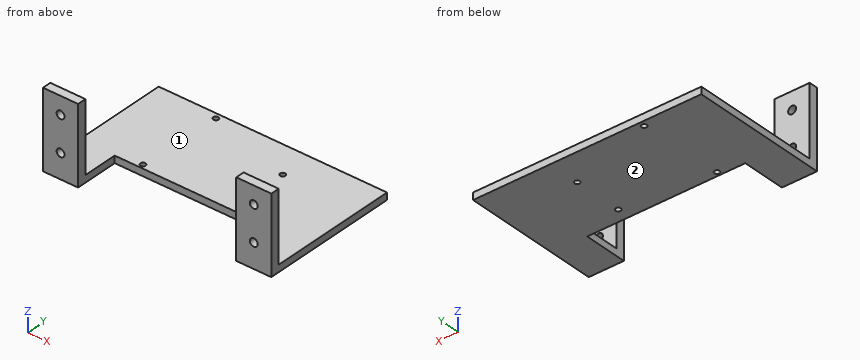
from build123d import *

# Parameters (mm, degrees)
SKETCH1_W                 = 20
SKETCH1_H                 = 44
SKETCH1_R                 = 2.25
BOSS_EXTRUDE1_DEPTH       = 5
BOSS_EXTRUDE1_2_DEPTH     = 5
SKETCH2_W                 = 130.04
SKETCH2_H                 = 4
BOSS_EXTRUDE2_DEPTH       = 74
BOSS_EXTRUDE2_DEPTH_BACK  = 5
SKETCH3_W                 = 90.04
SKETCH3_H                 = 25
CUT_EXTRUDE1_DEPTH        = 5
F_3_0MM_DOWEL_HOLE1_D     = 3
F_3_0MM_DOWEL_HOLE1_DEPTH = 5
F_3_0MM_DOWEL_HOLE1_TIP   = 0.901290929


with BuildPart() as part:
    # Sketch1 → Boss-Extrude1 (new body)
    with BuildSketch(Plane(origin=(0, 0, 0), x_dir=(1, 0, 0), z_dir=(0, 1, 0))):
        with Locations((0, 12)):
            Rectangle(SKETCH1_W, SKETCH1_H)
        Circle(SKETCH1_R, mode=Mode.SUBTRACT)
        with Locations((0, 20)):
            Circle(SKETCH1_R, mode=Mode.SUBTRACT)
    extrude(amount=BOSS_EXTRUDE1_DEPTH)



with BuildPart() as body_2:
    # Sketch1 → Boss-Extrude1 2 (new body)
    with BuildSketch(Plane(origin=(0, 0, 0), x_dir=(1, 0, 0), z_dir=(0, 1, 0))):
        with Locations((110.04, 12)):
            Rectangle(SKETCH1_W, SKETCH1_H)
        with Locations((110.04, 20)):
            Circle(SKETCH1_R, mode=Mode.SUBTRACT)
        with Locations((110.04, 0)):
            Circle(SKETCH1_R, mode=Mode.SUBTRACT)
    extrude(amount=BOSS_EXTRUDE1_2_DEPTH)


with BuildPart() as part_1:
    add(part.part)

    add(body_2.part)  # Boss-Extrude2 merges body 2
    # Sketch2 → Boss-Extrude2 (add, two sides)
    with BuildSketch(Plane(origin=(0, 5, 0), x_dir=(1, 0, 0), z_dir=(0, 1, 0))) as boss_extrude2_sk:
        with Locations((55.02, 32)):
            Rectangle(SKETCH2_W, SKETCH2_H)
    extrude(amount=BOSS_EXTRUDE2_DEPTH)
    extrude(boss_extrude2_sk.sketch, amount=-BOSS_EXTRUDE2_DEPTH_BACK)

    # Sketch3 → Cut-Extrude1 (cut)
    with BuildSketch(Plane.XY.offset(-30)):
        with Locations((55.02, 12.5)):
            Rectangle(SKETCH3_W, SKETCH3_H)
    extrude(amount=-CUT_EXTRUDE1_DEPTH, mode=Mode.SUBTRACT)

    # Ø3.0mm Dowel Hole1
    with Locations(Plane(origin=(55.834419791, -56, -30), x_dir=(1, 0, 0), z_dir=(0, 0, 1))):
        with Locations((-30.594419791, 131.8), (20.205580209, 116.56), (20.205580209, 88.62), (-31.864419791, 83.54)):
            Hole(F_3_0MM_DOWEL_HOLE1_D / 2, depth=F_3_0MM_DOWEL_HOLE1_DEPTH)
            with Locations((0, 0, -(F_3_0MM_DOWEL_HOLE1_DEPTH + F_3_0MM_DOWEL_HOLE1_TIP / 2))):  # 118° drill point
                Cone(0, F_3_0MM_DOWEL_HOLE1_D / 2, F_3_0MM_DOWEL_HOLE1_TIP, mode=Mode.SUBTRACT)


solid = part_1.part
The listing builds one solid part. Answer for the finished solid, in the listing's coordinates (mm). Face numbers are marked on the shaded views. A direction names the side the tool comes from. Coordinates: 2 decimals unless noted, no trailing zeros. Order: outer loops, then holes, each group sorted by start corner. A loop starts at its lowest first (then second) coordinate and runs counter-clockwise, first axis right, second up. Notation, with made-up numbers: M 62,-37.5 L 72,-37.5 A14 cw 72,-17.5 Z; hole C -10,-17.75 d10. An arc over 180 degrees is marked long. Use CSV: the item, a comma, the result in double quotes.
Q1. A tool of negligible diameter and unlimited length cuts with its end or side. For the marked faces 1 and 2, from which of +Z, -Z, +X, -X, +Y, -Y can it reach the whole face along a straight path? Write none if from no direction.
Here are the results:
face 1,"+Z, +X, -X, +Y"
face 2,"-Z, +X, -X, +Y, -Y"
Q2. Section B-B (x = 76.04) is taken. Determine the outline of the cut face in (y, z).
Here are the results:
outline,"M 25,-34 L 31.12,-34 L 31.12,-30 L 25,-30 Z; M 34.12,-34 L 59.06,-34 L 59.06,-30 L 34.12,-30 Z; M 62.06,-34 L 79,-34 L 79,-30 L 62.06,-30 Z"
Q3. Given pin 1 Ø3.5 at (x, y) = (76.04, 32.62) entering from +Z; pin 2 Ø3 at (x, z) = (60.5, -31.5) entering from -Y; pin 3 Ø3.5 at (x, z) = (110.04, -20) entering from +Y; pin 4 Ø10 at (x, z) = (-1.5, -2.5) entering from +Y, each flat-ended and moving along its own axis, determine where each tip first touches the part or whether it passes through.
Here are the results:
pin 1,"z = -30"
pin 2,"y = 25"
pin 3,"through"
pin 4,"y = 5"
Q4. Straight lines are drawn through the part: L1, parallel to Z at x = 0, y = 1.25; L2, parallel to X at y = 2.9, z = -20; L3, parallel to Y at x = 25, z = -31. For each, find the intervals that lie inside material, in ascending order.
Here are the results:
L1,"-34 to -22.25, -17.75 to -2.25, 2.25 to 10"
L2,"-10 to -2.25, 2.25 to 10, 100.04 to 107.79, 112.29 to 120.04"
L3,"25 to 26.45, 28.63 to 74.32, 77.28 to 79"
Q5. Section C-C (z = -20) is taken. Determine the outline of the cut face in (x, y), then the cut area to 3 significant figures.
Here are the results:
outline,"M -10,0 L -2.25,0 L -2.25,5 L -10,5 Z; M 2.25,0 L 10,0 L 10,5 L 2.25,5 Z; M 100.04,0 L 107.79,0 L 107.79,5 L 100.04,5 Z; M 112.29,0 L 120.04,0 L 120.04,5 L 112.29,5 Z"
area,"155 mm2"
Q6. Section A-A (y = 23.5) is taken. Determine the outline of the cut face in (x, z).
Here are the results:
outline,"M -10,-34 L 10,-34 L 10,-30 L -10,-30 Z; M 100.04,-34 L 120.04,-34 L 120.04,-30 L 100.04,-30 Z"
Q7. Section D-D (z = -7) is taken. Determine the outline of the cut face in (x, y).
Here are the results:
outline,"M -10,0 L 10,0 L 10,5 L -10,5 Z; M 100.04,0 L 120.04,0 L 120.04,5 L 100.04,5 Z"
